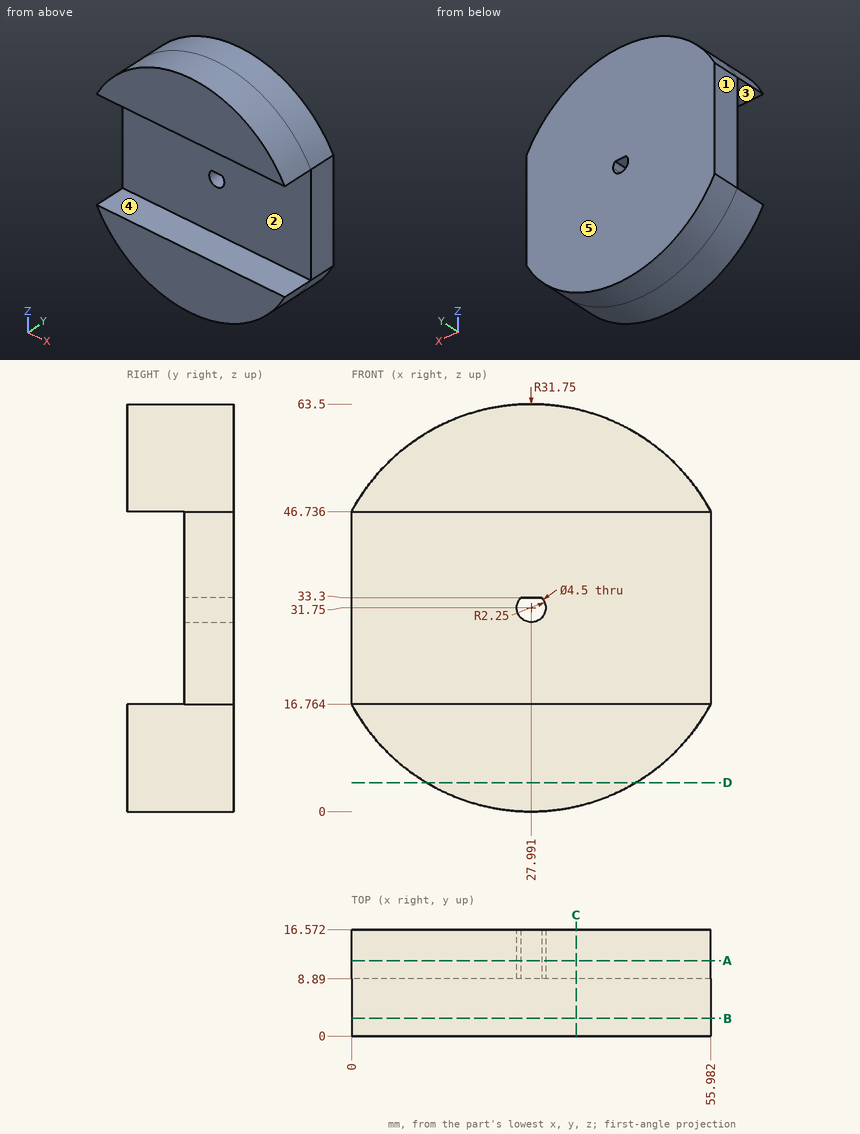
Source: three-view drawing plus pictorial views. Frame: mm from the lowest corner of the part. A direction names the side the tool comes from. Round coordinates to 2 decimals unless told otherwise and drop trailing zeros. Order: outer loops, then holes, each group sorted by start corner. A loop starts at its lowest first (then second) coordinate and runs counter-clockwise, first axis right, second up. Notation, with made-up numbers: (27.25, 88.25) -> (33.25, 88.25) arc R14 cw to (33.25, 115.25) -> close; hole circle Ø8 at (76.5, 85). An arc over 180 degrees is marked (long way). Use one line per item in the form item = value. Start each with the question number.
1. Line query: probe 1 along Y at (x, z) = (28, 42.5); probe 2 along Z at (x, y) = (44, 6.75) (1 decimal); probe 3 along Z at (x, y) = (46.5, 2.75) (1 decimal). Output: solid intervals per line, ascending.
2. Reachability of the marked faces 4 and 5 from +Z, -Z, +X, -X, +Y, -Y: full face, straight path, thin tool, end or side. Return the list, or none.
3. Pin query (flat end, axial travel): pin 1 Ø4.5 at (x, y) = (42, 6) entering from -Z; pin 2 Ø6 at (x, z) = (27.99, 31.75) entering from -Y; pin 3 Ø3 at (x, y) = (20.5, 6.5) entering from +Z. Return the tip coordinate at first contact, or that it passes through.
4. Cut plane D-D (z = 4.5). Return the cut outline in (x, y) (1 decimal).
5. Cut plane C-C (x = 35). Return the cut outline in (y, z), then the cut area to 3 significant figures.
6. Cut plane A-A (y = 11.75). Return the cut outline in (x, z), then the cut area to 3 significant figures.
7. Cut plane B-B (y = 2.75). Return the cut outline in (x, z), then the cut area to 3 significant figures.
8. Draft query along Z for the marked faces 1, 2 and 3. Return one class per face: pulls with the +Z half, pulls with the -Z half, needs draft (parallel to the pull), parting line crosses it, or undercut.
Solution:
q1.probe_1 = 8.89 to 16.57
q1.probe_2 = 4.3 to 16.8, 46.7 to 59.2
q1.probe_3 = 6 to 16.8, 46.7 to 57.5
q2.face_4 = +X, -X, -Y
q2.face_5 = +Z, -Z, +X, -X, +Y
q3.pin_1 = 2.26
q3.pin_2 = 8.89
q3.pin_3 = 62.93
q4.outline = (11.7, 0) -> (44.3, 0) -> (44.3, 16.6) -> (11.7, 16.6) -> close
q5.outline = (0, 0.78) -> (16.57, 0.78) -> (16.57, 62.72) -> (0, 62.72) -> (0, 46.74) -> (8.89, 46.74) -> (8.89, 16.76) -> (0, 16.76) -> close
q5.area = 760 mm^2
q6.outline = (0, 16.76) arc R31.75 ccw to (55.98, 16.76) -> (55.98, 46.74) arc R31.75 ccw to (0, 46.74) -> close; hole (26.36, 33.3) arc R2.25 ccw (long way) to (29.62, 33.3) -> close
q6.area = 3,000 mm^2
q7.outline = (0, 16.76) arc R31.75 ccw to (55.98, 16.76) -> close; (0, 46.74) -> (55.98, 46.74) arc R31.75 ccw to start
q7.area = 1,340 mm^2
q8.face_1 = needs draft
q8.face_2 = undercut
q8.face_3 = undercut
